Check sheet for the modelled part. Datum: model origin and axes. Units: mm. Face numbers are marked on the shaded views. A direction names the side the tool comes from. Round coordinates to 2 decimals unless told otherwise and drop trailing zeros. Loops run counter-clockwise (first coordinate to the right, second up) from the corner with the lowest first, then second, coordinate; pieces in that order, holes last. Notation, with made-up numbers: M 53,44.5 L 76,44.5 A20 cw 76,63.5 Z; hole C 77.5,-5 d2. An arc over 180 degrees is marked long. Write item = value, one per line. Start each with the question number.
(1) Go/stop test with flat-tipped pins: P1, Ø8, axis at x = 14, z = -4.5, coming from the -Y side (3 decimals); P2, Ø8, axis at y = -16.67, z = -22.22, coming from the +X side. Record where each tip stops, or that it passes through.
(2) Cross-section at A-A on y = -27. Record the boundary of the cut face in (x, z) (1 decimal), plus the area to 3 significant figures.
(3) Set-up check for the marked faces 1 and 2: record each of +Z, -Z, +X, -X, +Y, -Y from which the full face is reachable in a straight line by a thin tool's end or side.
(4) Cross-section at D-D on y = -15.5. Record the boundary of the cut face in (x, z) (1 decimal).
(5) Scan lines: L1, parallel to Z at x = 19, y = -25 (3 decimals); L2, parallel to X at y = -28, z = -6; L3, parallel to Y at x = 17, z = 10 (3 decimals). Record each from-to range of solid material in increasing order. Write a range as from..to.
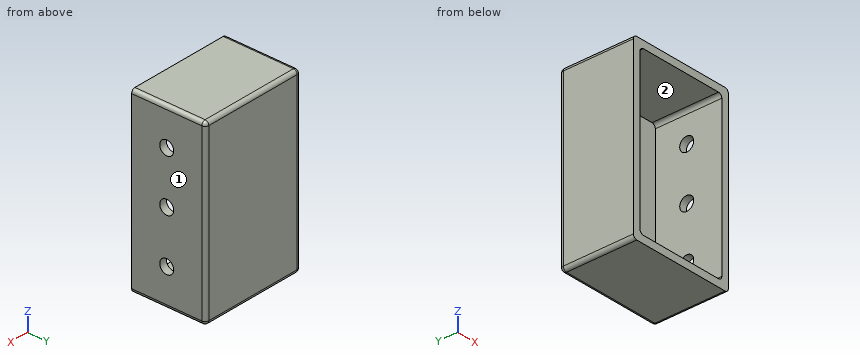
from build123d import *

# Parameters (mm, degrees)
F0_W     = 45.72
F0_H     = 76.2
F0_W_2   = 39.37
F0_H_2   = 69.85
F1_DEPTH = 31.75
F2_R     = 1.5875
F4_DEPTH = 3.175
F5_R     = 1.5875
F3_R     = 3
F6_DEPTH = 3.175


with BuildPart() as f1:
    # F0 (on Front) → F1 (new body)
    with BuildSketch(Plane.XZ):
        with Locations((1.461808, 0)):
            Rectangle(F0_W, F0_H)
        with Locations((1.461808, 0)):
            Rectangle(F0_W_2, F0_H_2, mode=Mode.SUBTRACT)
    extrude(amount=F1_DEPTH)

    # F2
    f2_edges = [f1.edges().sort_by_distance(p)[0] for p in [
        (24.321808, -15.875, -38.1),
        (24.321808, -15.875, 38.1),
        (-21.398192, -15.875, 38.1),
        (-21.398192, -15.875, -38.1),
        (-21.398192, 0, 0),
        (1.461808, 0, -38.1),
        (24.321808, 0, 0),
        (1.461808, 0, 38.1),
    ]]
    fillet(f2_edges, radius=F2_R)

    # F0 (on Front) → F4 (join)
    with BuildSketch(Plane.XZ):
        with Locations((1.461808, 0)):
            Rectangle(F0_W_2, F0_H_2)
    extrude(amount=F4_DEPTH)

    # F5
    f5_edges = [f1.edges().sort_by_distance(p)[0] for p in [
        (-18.223192, -17.4625, -34.925),
        (-18.223192, -17.4625, 34.925),
        (21.146808, -17.4625, -34.925),
        (21.146808, -17.4625, 34.925),
    ]]
    fillet(f5_edges, radius=F5_R)

    # F3 (on face) → F6 (cut, through all)
    with BuildSketch(Plane.YZ.offset(24.321808)):
        with Locations((-16.66875, -22.225)):
            Circle(F3_R)
        with Locations((-16.66875, 0)):
            Circle(F3_R)
        with Locations((-16.66875, 22.225)):
            Circle(F3_R)
    extrude(amount=-F6_DEPTH, mode=Mode.SUBTRACT)


solid = f1.part
Result:
q1.P1 = -3.175
q1.P2 = 24.32
q2.outline = M -21.4,-36.5 A1.6 ccw -19.8,-38.1 L 22.7,-38.1 A1.6 ccw 24.3,-36.5 L 24.3,36.5 A1.6 ccw 22.7,38.1 L -19.8,38.1 A1.6 ccw -21.4,36.5 Z; hole M -18.2,-33.3 A1.6 ccw -16.6,-34.9 L 19.6,-34.9 A1.6 ccw 21.1,-33.3 L 21.1,33.3 A1.6 ccw 19.6,34.9 L -16.6,34.9 A1.6 ccw -18.2,33.3 Z
q2.area = 734 mm^2
q3.face_1 = +Z, -Z, +X, +Y, -Y
q3.face_2 = -Y
q4.outline = M -21.4,-36.5 A1.6 ccw -19.8,-38.1 L 22.7,-38.1 A1.6 ccw 24.3,-36.5 L 24.3,-25 L 21.1,-25 L 21.1,-33.3 A1.6 cw 19.6,-34.9 L -16.6,-34.9 A1.6 cw -18.2,-33.3 L -18.2,33.3 A1.6 cw -16.6,34.9 L 19.6,34.9 A1.6 cw 21.1,33.3 L 21.1,25 L 24.3,25 L 24.3,36.5 A1.6 ccw 22.7,38.1 L -19.8,38.1 A1.6 ccw -21.4,36.5 Z; M 21.1,-19.5 L 24.3,-19.5 L 24.3,-2.8 L 21.1,-2.8 Z; M 21.1,2.8 L 24.3,2.8 L 24.3,19.5 L 21.1,19.5 Z
q5.L1 = -38.1..-34.925, 34.925..38.1
q5.L2 = -21.4..-18.22, 21.15..24.32
q5.L3 = -3.175..0
